```python
from build123d import *

# Parameters (mm, degrees)
SKETCH1_R                        = 76.1746
BOSS_EXTRUDE1_DEPTH              = 3.175
SKETCH3_R                        = 73.3171
BOSS_EXTRUDE2_DEPTH              = 3.175
F_97_0_0059_DIAMETER_HOLE1_D     = 6.985
F_97_0_0059_DIAMETER_HOLE1_DEPTH = 10.0076
F_97_0_0059_DIAMETER_HOLE1_TIP   = 2.016395815
SKETCH9_R                        = 1.292031205
SKETCH9_W                        = 51.054
SKETCH9_H                        = 12.954
CUT_EXTRUDE1_DEPTH               = 108.914141197
SKETCH11_R                       = 2.159
CUT_EXTRUDE3_DEPTH               = 108.914141197
CIRPATTERN2_COUNT                = 3
SKETCH15_R                       = 4.7625
CUT_EXTRUDE4_DEPTH               = 6.35
HOLE1_D                          = 3.2639
CIRPATTERN3_COUNT                = 3
CIRPATTERN3_ANGLE                = 240
CIRPATTERN4_COUNT                = 2
CIRPATTERN4_ANGLE                = 120


with BuildPart() as part:
    # Sketch1 → Boss-Extrude1 (new body)
    with BuildSketch(Plane(origin=(0, 0, 0), x_dir=(1, 0, 0), z_dir=(0, 1, 0))):
        with Locations(Location((0, 0, 0), (0, 0, 270))):
            Circle(SKETCH1_R)
    extrude(amount=-BOSS_EXTRUDE1_DEPTH)

    # Sketch3 → Boss-Extrude2 (add)
    with BuildSketch(Plane.XZ.offset(3.175)):
        with Locations(Location((0, 0, 0), (0, 0, 270))):
            Circle(SKETCH3_R)
    extrude(amount=BOSS_EXTRUDE2_DEPTH)

    # #97 (0.0059) Diameter Hole1
    with Locations(Plane(origin=(0, -6.35, 0), x_dir=(-1, 0, 0), z_dir=(0, -1, 0))):
        with Locations((0, 0)):
            Hole(F_97_0_0059_DIAMETER_HOLE1_D / 2, depth=F_97_0_0059_DIAMETER_HOLE1_DEPTH)
            with Locations((0, 0, -(F_97_0_0059_DIAMETER_HOLE1_DEPTH + F_97_0_0059_DIAMETER_HOLE1_TIP / 2))):  # 120° drill point
                Cone(0, F_97_0_0059_DIAMETER_HOLE1_D / 2, F_97_0_0059_DIAMETER_HOLE1_TIP, mode=Mode.SUBTRACT)

    # Sketch8 → #97 (0.0059) Diameter Hole3 (revolve, cut)
    with BuildSketch(Plane(origin=(0, 0, -19.05), x_dir=(0, 0, 1), z_dir=(1, 0, 0))):
        Polygon((0, 0), (0, 11.892013544), (3.2639, 10.0076), (3.2639, 0), align=None)
    f_97_0_0059_diameter_hole3 = revolve(axis=Axis((0, 6.35, -19.05), (0, -1, 0)), mode=Mode.SUBTRACT)

    # Mirror1: #97 (0.0059) Diameter Hole3 across plane
    add(f_97_0_0059_diameter_hole3.mirror(Plane.XY), mode=Mode.SUBTRACT)

    # Sketch9 → Cut-Extrude1 (cut, through all)
    with BuildSketch(Plane(origin=(0, 0, 0), x_dir=(1, 0, 0), z_dir=(0, 1, 0))):
        with Locations(Location((-1.1176, -66.421, 0), (0, 0, 270))):
            Circle(SKETCH9_R)
        with Locations(Location((-1.1176, -45.847, 0), (0, 0, 90))):
            Circle(SKETCH9_R)
        with Locations((-1.1176, -56.134)):
            Rectangle(SKETCH9_W, SKETCH9_H)
    cut_extrude1 = extrude(amount=-CUT_EXTRUDE1_DEPTH, mode=Mode.SUBTRACT)

    # Sketch11 → Cut-Extrude3 (cut, symmetric)
    with BuildSketch(Plane(origin=(0, 0, 0), x_dir=(1, 0, 0), z_dir=(0, 1, 0))):
        with Locations(Location((28.575, 49.493351826, 0), (0, 0, 270))):
            Circle(SKETCH11_R)
    cut_extrude3 = extrude(amount=CUT_EXTRUDE3_DEPTH, both=True, mode=Mode.SUBTRACT)

    # CirPattern2: Cut-Extrude3 ×3 about axis
    cirpattern2_axis = Axis((0, 0, 0), (0, 1, 0))
    for i in range(1, CIRPATTERN2_COUNT):
        add(cut_extrude3.rotate(cirpattern2_axis, i * 360 / CIRPATTERN2_COUNT), mode=Mode.SUBTRACT)

    # Sketch15 → Cut-Extrude4 (cut)
    with BuildSketch(Plane(origin=(0, 0, 0), x_dir=(1, 0, 0), z_dir=(0, 1, 0))):
        with Locations(Location((-42.7800008, 4.89000038, 0), (0, 0, 270))):
            Circle(SKETCH15_R)
        with Locations(Location((22.86, -41.1899989, 0), (0, 0, 270))):
            Circle(SKETCH15_R)
    extrude(amount=-CUT_EXTRUDE4_DEPTH, mode=Mode.SUBTRACT)

    # Hole1 (through all)
    with Locations(Plane(origin=(0, 0, 0), x_dir=(1, 0, 0), z_dir=(0, 1, 0))):
        with Locations((0, 58.07456)):
            hole1 = Hole(HOLE1_D / 2)

    # CirPattern3: Hole1 ×3 about axis
    cirpattern3_axis = Axis((0, 0, 0), (0, 1, 0))
    for i in range(1, CIRPATTERN3_COUNT):
        add(hole1.rotate(cirpattern3_axis, i * CIRPATTERN3_ANGLE / (CIRPATTERN3_COUNT - 1)), mode=Mode.SUBTRACT)

    # CirPattern4: Cut-Extrude1 ×2 about axis
    cirpattern4_axis = Axis((0, 0, 0), (0, 1, 0))
    for i in range(1, CIRPATTERN4_COUNT):
        add(cut_extrude1.rotate(cirpattern4_axis, i * CIRPATTERN4_ANGLE / (CIRPATTERN4_COUNT - 1)), mode=Mode.SUBTRACT)


solid = part.part
```
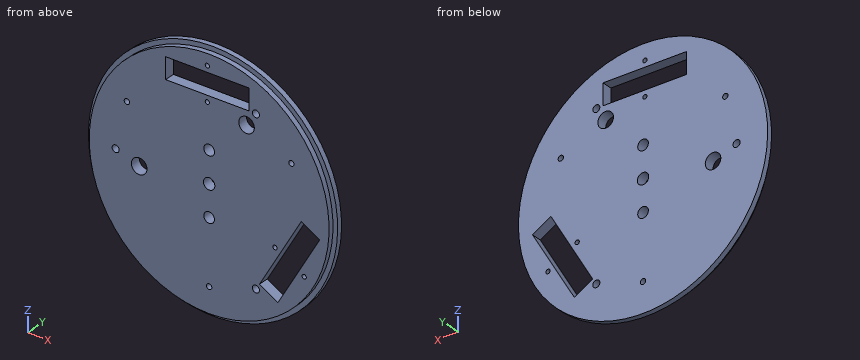
The model under review builds one solid part; all positions refer to its coordinate system, in mm. Round coordinates to 2 decimals unless told otherwise and drop trailing zeros. Loops run counter-clockwise (first coordinate to the right, second up) from the corner with the lowest first, then second, coordinate; pieces in that order, holes last.
Item 1: For line 1 (X direction, y = -1.75, z = -4.89); line 2 (X direction, y = -5.5, z = -48); line 3 (Z direction, x = 41, y = -2.5), list the stretches that pass through material, from the lowest coordinate up.
Determined:
line 1: x = -76.02 to -47.54, -38.02 to 54.52, 61.76 to 76.02
line 2: x = -55.42 to 27.02, 30.13 to 34.32, 44.58 to 55.42
line 3: z = -64.2 to -51.86, -28.3 to -23.02, -20.89 to 64.2
Item 2: Take a section at D-D (y = -2). Give the number of separate pieces and of enclosed holes in the cut face, then the cut area to 3 significant figures.
Determined:
separate pieces: 1
enclosed holes: 17
area: 16,600 mm2
Item 3: Clearance check with flat-ended pins moving along their axes: pin 1 Ø2 at (x, z) = (0, -58.07) entering from -Y; pin 2 Ø3 at (y, z) = (-1.5, 54) entering from -X; pin 3 Ø3 at (x, y) = (-9.5, -4.5) entering from +Z; pin 4 Ø3 at (y, z) = (-1, -37) entering from +X. State where each tip first meets the part, or that it passes through.
Determined:
pin 1: passes through
pin 2: stops at x = -55.19
pin 3: stops at z = 75.66
pin 4: stops at x = 67.4
Item 4: Take a section at C-C (z = 19.05). Write out the cut boundary in (x, y) (3 decimals), then the cut area to 3 significant figures.
Determined:
outline: (-73.754, -3.175) - (-70.799, -3.175) - (-70.799, -6.35) - (-3.264, -6.35) - (-3.264, 0) - (-73.754, 0) - close; (3.264, -6.35) - (70.799, -6.35) - (70.799, -3.175) - (73.754, -3.175) - (73.754, 0) - (3.264, 0) - close
area: 876 mm2
Item 5: Take a section at B-B (x = 21). Write out the cut boundary in (y, z) (3 decimals).
Determined:
outline: (-6.35, -70.245) - (-3.175, -70.245) - (-3.175, -73.223) - (0, -73.223) - (0, 36.806) - (-6.35, 36.806) - close; (-6.35, 45.574) - (0, 45.574) - (0, 49.657) - (-6.35, 49.657) - close; (-6.35, 62.611) - (0, 62.611) - (0, 73.223) - (-3.175, 73.223) - (-3.175, 70.245) - (-6.35, 70.245) - close
